```python
from build123d import *

# Parameters (mm, degrees)
F0_R     = 30.48
F0_R_2   = 2.921
F0_R_3   = 2.032
F1_DEPTH = 2.54
F2_R     = 20.32
F2_R_2   = 17.78
F3_DEPTH = 5.08
F5_DEPTH = 5.08


with BuildPart() as f1:
    # F0 (on Top) → F1 (new body)
    with BuildSketch(Plane.XY):
        Circle(F0_R)
        with BuildLine():
            ThreePointArc((2.921, -9.779), (-2.0654589078, -11.8444589078), (0, -6.858))
            ThreePointArc((0, -6.858), (2.0654589078, -7.7135410922), (2.921, -9.779))
        make_face(mode=Mode.SUBTRACT)
        with Locations((-9.779, 0)):
            Circle(F0_R_2, mode=Mode.SUBTRACT)
        with BuildLine():
            ThreePointArc((0, 6.35), (4.4901280605, 4.4901280605), (6.35, 0))
            ThreePointArc((6.35, 0), (4.4901280605, -4.4901280605), (0, -6.35))
            ThreePointArc((0, -6.35), (-4.4901280605, -4.4901280605), (-6.35, 0))
            ThreePointArc((-6.35, 0), (-4.4901280605, 4.4901280605), (0, 6.35))
        make_face(mode=Mode.SUBTRACT)
        with BuildLine():
            ThreePointArc((12.7, 0), (9.779, -2.921), (6.858, 0))
            ThreePointArc((6.858, 0), (9.779, 2.921), (12.7, 0))
        make_face(mode=Mode.SUBTRACT)
        with BuildLine():
            ThreePointArc((2.921, 9.779), (2.0654589078, 7.7135410922), (0, 6.858))
            ThreePointArc((0, 6.858), (-2.0654589078, 11.8444589078), (2.921, 9.779))
        make_face(mode=Mode.SUBTRACT)
        with BuildLine():
            ThreePointArc((2.921, 9.779), (-2.0654589078, 11.8444589078), (0, 6.858))
            ThreePointArc((0, 6.858), (2.0654589078, 7.7135410922), (2.921, 9.779))
        make_face()
        with BuildLine():
            ThreePointArc((2.032, 9.779), (1.4368409794, 8.3421590206), (0, 7.747))
            ThreePointArc((0, 7.747), (-1.4368409794, 11.2158409794), (2.032, 9.779))
        make_face(mode=Mode.SUBTRACT)
        with Locations((-9.779, 0)):
            Circle(F0_R_2)
        with Locations((-9.779, 0)):
            Circle(F0_R_3, mode=Mode.SUBTRACT)
        with BuildLine():
            ThreePointArc((2.921, -9.779), (2.0654589078, -7.7135410922), (0, -6.858))
            ThreePointArc((0, -6.858), (-2.0654589078, -11.8444589078), (2.921, -9.779))
        make_face()
        with BuildLine():
            ThreePointArc((2.032, -9.779), (-1.4368409794, -11.2158409794), (0, -7.747))
            ThreePointArc((0, -7.747), (1.4368409794, -8.3421590206), (2.032, -9.779))
        make_face(mode=Mode.SUBTRACT)
        with BuildLine():
            ThreePointArc((12.7, 0), (9.779, 2.921), (6.858, 0))
            ThreePointArc((6.858, 0), (9.779, -2.921), (12.7, 0))
        make_face()
        with BuildLine():
            ThreePointArc((11.811, 0), (9.779, -2.032), (7.747, 0))
            ThreePointArc((7.747, 0), (9.779, 2.032), (11.811, 0))
        make_face(mode=Mode.SUBTRACT)
    extrude(amount=F1_DEPTH)

    # F2 (on face) → F3 (join)
    with BuildSketch(Plane(origin=(0, 0, 0), x_dir=(1, 0, 0), z_dir=(0, 0, -1))):
        Circle(F2_R)
        Circle(F2_R_2, mode=Mode.SUBTRACT)
    extrude(amount=F3_DEPTH)

    # F4 (on face) → F5 (cut)
    with BuildSketch(Plane(origin=(0, 0, -5.08), x_dir=(1, 0, 0), z_dir=(0, 0, -1))):
        with BuildLine():
            Line((6.8041114275, 16.4265780881), (7.7761273457, 18.7732321006))
            ThreePointArc((7.7761273457, 18.7732321006), (3.9642353434, 19.9295568978), (0, 20.32))
            Line((0, 20.32), (0, 17.78))
            ThreePointArc((0, 17.78), (3.4687059254, 17.4383622856), (6.8041114275, 16.4265780881))
        make_face()
    extrude(amount=-F5_DEPTH, mode=Mode.SUBTRACT)


solid = f1.part
```
Work out the finished part from the listing and answer in its coordinate system (mm). A direction names the side the tool comes from. Coordinates: 2 decimals unless noted, no trailing zeros. Loops run counter-clockwise (first coordinate to the right, second up) from the corner with the lowest first, then second, coordinate; pieces in that order, holes last.
1) Section A-A (z = 1) is taken. Give the vertices of the cut face in (x, y), plus the area to 3 significant figures.
Results:
outline: circle Ø60.96 at (0, 0); hole circle Ø4.06 at (-9.78, 0); hole circle Ø12.7 at (0, 0); hole circle Ø4.06 at (0, -9.78); hole circle Ø4.06 at (0, 9.78); hole circle Ø4.06 at (9.78, 0)
area: 2,740 mm2
2) For faces 4 (the cylindrical face through (-4.78, 19.75, -2.5)), 5 (the flat face through (0, -19, -3)), 6 (the flat face through (-7, 0, 2.54)), determine the directions among +Z, -Z, +X, -X, +Y, -Y from which every point of the face is accessible in a straight line to the end or side of a thin tool.
Results:
face 4: -Z
face 5: -Z, -Y
face 6: +Z, +X, -X, +Y, -Y
3) Consider probe 1 along X at (y, z) = (-1, 1.5); probe 2 along X at (y, z) = (0, -2.45); probe 3 along Z at (x, y) = (-15, -20.5). Determine where each line is inside the solid, lowest interval first.
Results:
probe 1: x = -30.46 to -11.55, -8.01 to -6.27, 6.27 to 8.01, 11.55 to 30.46
probe 2: x = -20.32 to -17.78, 17.78 to 20.32
probe 3: z = 0 to 2.54
4) Section C-C (x = 19) is taken. Give the vertices of the cut face in (y, z).
Results:
outline: (-23.83, 0) - (-7.2, 0) - (-7.2, -5.08) - (7.2, -5.08) - (7.2, 0) - (23.83, 0) - (23.83, 2.54) - (-23.83, 2.54) - close
5) Flat-ended cylindrical pins translate along their axes: pin 1 (1.5 mm diameter, centred on x = 16.5, y = -23, fed in from -Z); pin 2 (1.3 mm diameter, centred on y = -19, z = -2.5, fed in from +X); pin 3 (2 mm diameter, centred on x = -12, z = -1.5, fed in from -Y); pin 4 (3.5 mm diameter, centred on x = 0, y = -9.779, fed in from -Z). Find the tip coordinate at first contact, or state that the pin passes through.
Results:
pin 1: stops at z = 0
pin 2: stops at x = 8.73
pin 3: stops at y = -17.09
pin 4: passes through
6) For a pull along Y with two mould halves and no side action, classify faces 1 (the cylindrical face through (-4.18, 17.28, -2.5)), 2 (the cylindrical face through (-6.607, -29.755, 1.252)), 3 (the flat face through (7.28, -17.58, -2.58)) as +Y half, -Y half, draft (parallel to the pull), parting line (faces both ways), or undercut.
Results:
face 1: undercut
face 2: parting line
face 3: -Y half
7) Section B-B (y = -3) is taken. Give the vertices of the cut face in (x, z), plus the area to 3 significant figures.
Results:
outline: (-30.33, 0) - (-20.1, 0) - (-20.1, -5.08) - (-17.53, -5.08) - (-17.53, 0) - (-5.6, 0) - (-5.6, 2.54) - (-30.33, 2.54) - close; (5.6, 0) - (17.53, 0) - (17.53, -5.08) - (20.1, -5.08) - (20.1, 0) - (30.33, 0) - (30.33, 2.54) - (5.6, 2.54) - close
area: 152 mm2
